Could you check a few things on this model? Use its own coordinates, in mm. Face numbers are marked on the shaded views. A direction names the side the tool comes from. Give positions to 0.01 mm unless a question says otherwise; leave off trailing zeros. Write each loop counter-clockwise with the first axis right and the second up, starting at its lowest first coordinate (ties: lowest second). Pieces come first, ordered by that corner, then holes. Notation, with made-up numbers: (8.5, 68) - (42.5, 68) arc R20 ccw to (42.5, 96) - close; hole circle Ø10 at (75, 66.5). An arc over 180 degrees is marked (long way). Answer in a Markdown table with one row per item.
from build123d import *

# Parameters (mm, degrees)
SKETCH1_R           = 27.5
BOSS_EXTRUDE1_DEPTH = 27.5
SKETCH1_3_R         = 12
BOSS_EXTRUDE2_DEPTH = 17.5
CUT_EXTRUDE1_DEPTH  = 34
SKETCH3_R           = 17.5
SKETCH3_R_2         = 6
CUT_EXTRUDE2_DEPTH  = 34
CUT_EXTRUDE6_START  = 53
CUT_EXTRUDE6_DEPTH  = 53
SKETCH8_R           = 27.5
CUT_EXTRUDE7_DEPTH  = 47
SKETCH9_R           = 27.5
SKETCH9_R_2         = 17.5
BOSS_EXTRUDE3_DEPTH = 27.5


with BuildPart() as part:
    # Sketch1 → Boss-Extrude1 (new, symmetric)
    with BuildSketch(Plane.XY):
        Circle(SKETCH1_R)
    extrude(amount=BOSS_EXTRUDE1_DEPTH, both=True)

    # Sketch1_3 → Boss-Extrude2 (add, symmetric)
    with BuildSketch(Plane.XY):
        with BuildLine():
            Line((140.734972422, 11.925589642), (3.057732372, 27.329476262))
            ThreePointArc((3.057732372, 27.329476262), (20.498019907, 18.332517009), (27.5, 0))
            ThreePointArc((27.5, 0), (20.498019907, -18.332517009), (3.057732372, -27.329476262))
            Line((3.057732372, -27.329476262), (140.734972422, -11.925589642))
            ThreePointArc((140.734972422, -11.925589642), (127.400689205, 0), (140.734972422, 11.925589642))
        make_face()
        with Locations((139.400689205, 0)):
            Circle(SKETCH1_3_R)
    extrude(amount=BOSS_EXTRUDE2_DEPTH, both=True)

    # Sketch2 → Cut-Extrude1 (cut, symmetric)
    with BuildSketch(Plane(origin=(0, 0, 0), x_dir=(1, 0, 0), z_dir=(0, 1, 0))):
        Polygon((151.400689205, 17.5), (3.057732372, 17.5), (151.400689205, 9), align=None)
        Polygon((151.400689205, -9), (151.400689205, -17.5), (3.057732372, -17.5), align=None)
    extrude(amount=CUT_EXTRUDE1_DEPTH, both=True, mode=Mode.SUBTRACT)

    # Sketch3 → Cut-Extrude2 (cut, symmetric)
    with BuildSketch(Plane.XY):
        Circle(SKETCH3_R)
        with Locations((139.400689205, 0)):
            Circle(SKETCH3_R_2)
    extrude(amount=CUT_EXTRUDE2_DEPTH, both=True, mode=Mode.SUBTRACT)

    # Sketch7 → Cut-Extrude6 (cut)
    with BuildSketch(Plane.XY.offset(3.5).offset(CUT_EXTRUDE6_START)):
        with BuildLine():
            Line((36.413905406, 16.553775796), (129.115571862, 6.181938308))
            ThreePointArc((129.115571862, 6.181938308), (127.400689205, 0), (129.115571862, -6.181938308))
            Line((129.115571862, -6.181938308), (36.413905406, -16.553775796))
            ThreePointArc((36.413905406, -16.553775796), (40, 0), (36.413905406, 16.553775796))
        make_face()
    cut_extrude6 = extrude(amount=-CUT_EXTRUDE6_DEPTH, mode=Mode.SUBTRACT)

    # Mirror2: Cut-Extrude6 across plane
    add(cut_extrude6.mirror(Plane.XY), mode=Mode.SUBTRACT)

    # Sketch8 → Cut-Extrude7 (cut, symmetric)
    with BuildSketch(Plane.XY):
        Circle(SKETCH8_R)
    extrude(amount=CUT_EXTRUDE7_DEPTH, both=True, mode=Mode.SUBTRACT)

    # Sketch9 → Boss-Extrude3 (add, symmetric)
    with BuildSketch(Plane.XY):
        Circle(SKETCH9_R)
        Circle(SKETCH9_R_2, mode=Mode.SUBTRACT)
    extrude(amount=BOSS_EXTRUDE3_DEPTH, both=True)


solid = part.part
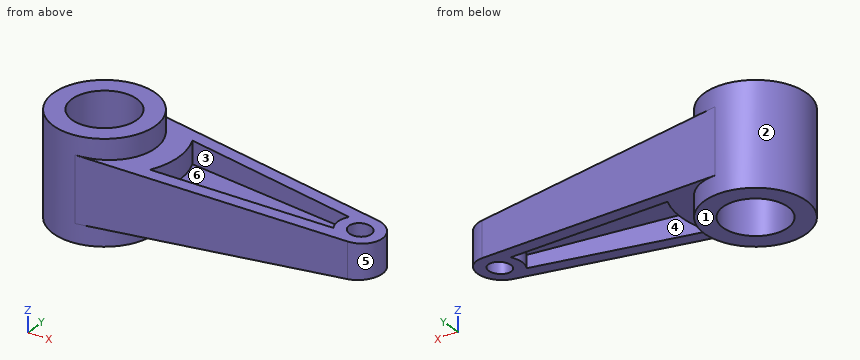
1) Imagine slicing it at C-C (z = -6.5). List the corners of the cut face in (x, y) for me, then the cut area to 3 significant figures.
Check values:
| item | result |
|---|---|
| outline | (3.06, -27.33) - (140.73, -11.93) arc R12 ccw to (140.73, 11.93) - (3.06, 27.33) arc R27.5 ccw (long way) to start; hole circle Ø35 at (0, 0); hole (36.41, -16.55) - (129.12, -6.18) arc R12 cw to (129.12, 6.18) - (36.41, 16.55) arc R40 cw to start; hole circle Ø12 at (139.4, 0) |
| area | 3,870 mm2 |
2) We'd pull the mould along Y, two halves only. Please class the marked faces 1, 2 and 3: +Y half, -Y half, draft (parallel to the pull), parting line (faces both ways), or undercut.
Check values:
| item | result |
|---|---|
| face 1 | draft |
| face 2 | parting line |
| face 3 | undercut |
3) If I drill on line 1 (Y direction, x = 0, z = -16); line 2 (X direction, y = -0.5, z = -8); line 3 (Y direction, x = -2, z = -6), over which ranges is the centre line in solid material (lowest first)?
Check values:
| item | result |
|---|---|
| line 1 | y = -27.5 to -17.5, 17.5 to 27.5 |
| line 2 | x = -27.5 to -17.49, 17.49 to 40, 127.41 to 133.42, 145.38 to 151.39 |
| line 3 | y = -27.43 to -17.39, 17.39 to 27.43 |
4) Imagine slicing it at B-B (x = 0). List the corners of the cut face in (y, z) for me, then the cut area to 3 significant figures.
Check values:
| item | result |
|---|---|
| outline | (-27.5, -27.5) - (-17.5, -27.5) - (-17.5, 27.5) - (-27.5, 27.5) - close; (17.5, -27.5) - (27.5, -27.5) - (27.5, 27.5) - (17.5, 27.5) - close |
| area | 1,100 mm2 |
5) Imagine slicing it at A-A (y = 0). List the corners of the cut face in (x, z) for me, then the cut area to 3 significant figures.
Check values:
| item | result |
|---|---|
| outline | (-27.5, -27.5) - (-17.5, -27.5) - (-17.5, 27.5) - (-27.5, 27.5) - close; (17.5, -27.5) - (27.5, -27.5) - (27.5, -16.1) - (40, -15.38) - (40, -3.5) - (127.4, -3.5) - (127.4, -10.38) - (133.4, -10.03) - (133.4, 10.03) - (127.4, 10.38) - (127.4, 3.5) - (40, 3.5) - (40, 15.38) - (27.5, 16.1) - (27.5, 27.5) - (17.5, 27.5) - close; (145.4, -9.34) - (151.4, -9) - (151.4, 9) - (145.4, 9.34) - close |
| area | 2,340 mm2 |
6) Will these pins go through, and if not, where does the flat tip stop? P1, Ø16.5, axis at x = 97.5, y = -1, coming from the +Z side; P2, Ø5, axis at x = 40, y = -19, coming from the +Z side; P3, Ø4, axis at y = 11.5, z = -20, coming from the +X side; P4, Ø10, axis at y = -5, z = -7.5, coming from the +X side.
Check values:
| item | result |
|---|---|
| P1 | stops at z = 3.5 |
| P2 | stops at z = 15.53 |
| P3 | stops at x = 25.81 |
| P4 | stops at x = 151.4 |
7) On a 3-axis mill with a long thin cutter (end or side, diameter ignored), from which of +Z, -Z, +X, -X, +Y, -Y can I reach the whole of each face in a straight line? I mean the marked faces 4, 5 and 6. Say none if no direction works.
Check values:
| item | result |
|---|---|
| face 4 | -Z |
| face 5 | +Z, -Z, +X |
| face 6 | +Z |
8) Imagine slicing it at D-D (y = 13.5). List the corners of the cut face in (x, z) for me, then the cut area to 3 significant figures.
Check values:
| item | result |
|---|---|
| outline | (-23.96, -27.5) - (-11.14, -27.5) - (-11.14, 27.5) - (-23.96, 27.5) - close; (11.14, -27.5) - (23.96, -27.5) - (23.96, -16.3) - (37.65, -15.52) - (37.65, -3.5) - (63.71, -3.5) - (63.71, -14.02) - (126.66, -10.42) - (126.66, 10.42) - (63.71, 14.02) - (63.71, 3.5) - (37.65, 3.5) - (37.65, 15.52) - (23.96, 16.3) - (23.96, 27.5) - (11.14, 27.5) - close |
| area | 3,570 mm2 |
